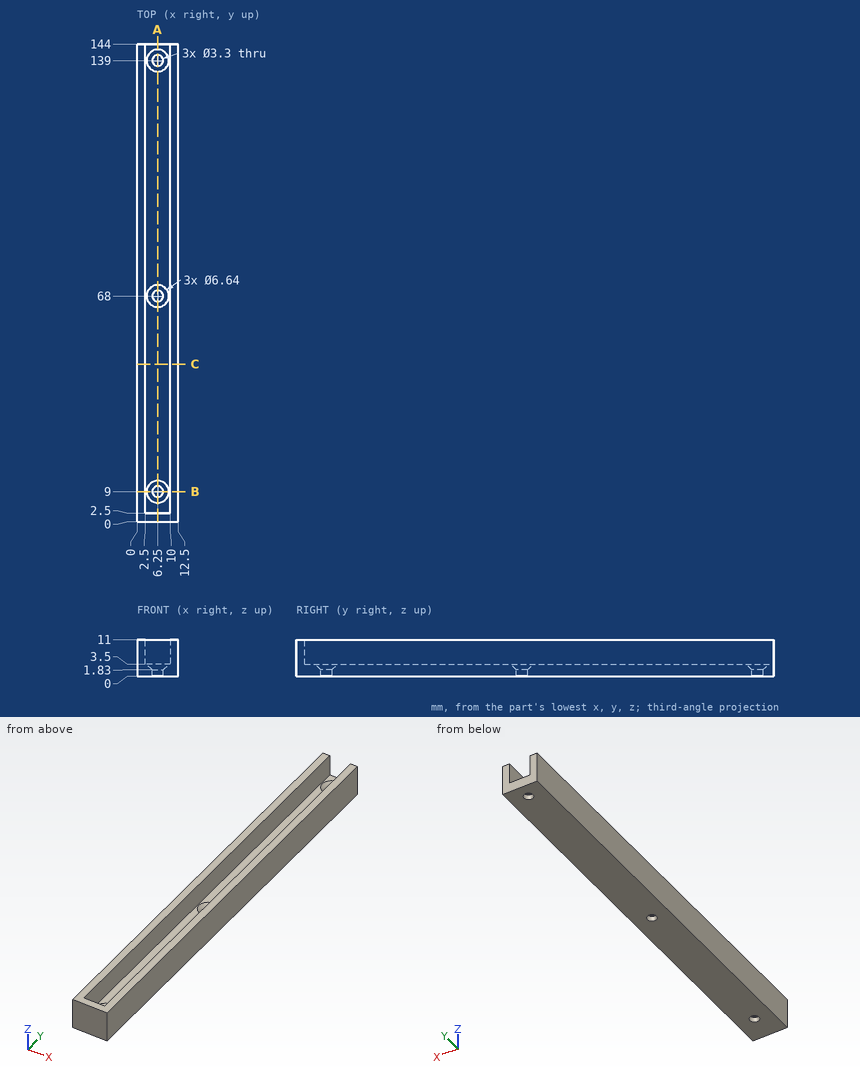
Drawing for the job (mm, zero at the part's lowest x, y, z). Give positions to 0.01 mm unless a question says otherwise; leave off trailing zeros. Write each loop counter-clockwise with the first axis right and the second up, starting at its lowest first coordinate (ties: lowest second). Pieces come first, ordered by that corner, then holes. Notation, with made-up numbers: (22, 0) -> (64, 0) arc R13 cw to (64, 5) -> close; hole circle Ø1 at (86.25, 87). An arc over 180 degrees is marked (long way). Put each result on its own line as item: value. Start each with the question number.
Item 1: Cut at A-A (x = 6.25). List the corners of the cut face in (y, z), then the cut area to 3 significant figures.
Item 2: Cut at B-B (y = 9). List the corners of the cut face in (x, z).
Item 3: Cut at C-C (y = 47.5). List the corners of the cut face in (x, z), then the cut area to 4 significant figures.
Item 4: Wall check: L1, parallel to Y at x = 6.25, z = 1.3; L2, parallel to X at y = 9, z = 1.1; L3, parallel to X at y = 59, z = 6.75. Give the ranges that are in metal, low to high. Write a range as [from, to].
Item 5: Pin check, flat tips, straight feed: pin 1 Ø6 at (x, z) = (6, 7.5) entering from +Y; pin 2 Ø3 at (x, z) = (4.5, 5) entering from -Y; pin 3 Ø4 at (x, y) = (5, 48) entering from +Z; pin 4 Ø2 at (x, y) = (6.25, 68) entering from -Z. Stop position of each tip, or through.
Answer list:
1. outline: (0, 0) -> (7.35, 0) -> (7.35, 1.83) -> (5.68, 3.5) -> (2.5, 3.5) -> (2.5, 11) -> (0, 11) -> close; (10.65, 0) -> (66.35, 0) -> (66.35, 1.83) -> (64.68, 3.5) -> (12.32, 3.5) -> (10.65, 1.83) -> close; (69.65, 0) -> (137.35, 0) -> (137.35, 1.83) -> (135.68, 3.5) -> (71.32, 3.5) -> (69.65, 1.83) -> close; (140.65, 0) -> (144, 0) -> (144, 3.5) -> (142.32, 3.5) -> (140.65, 1.83) -> close
1. area: 480 mm2
2. outline: (0, 0) -> (4.6, 0) -> (4.6, 1.83) -> (2.93, 3.5) -> (2.5, 3.5) -> (2.5, 11) -> (0, 11) -> close; (7.9, 0) -> (12.5, 0) -> (12.5, 11) -> (10, 11) -> (10, 3.5) -> (9.57, 3.5) -> (7.9, 1.83) -> close
3. outline: (0, 0) -> (12.5, 0) -> (12.5, 11) -> (10, 11) -> (10, 3.5) -> (2.5, 3.5) -> (2.5, 11) -> (0, 11) -> close
3. area: 81.25 mm2
4. L1: y = [0, 7.35], [10.65, 66.35], [69.65, 137.35], [140.65, 144]
4. L2: x = [0, 4.6], [7.9, 12.5]
4. L3: x = [0, 2.5], [10, 12.5]
5. pin 1: stops at y = 2.5
5. pin 2: stops at y = 0
5. pin 3: stops at z = 3.5
5. pin 4: passes through
